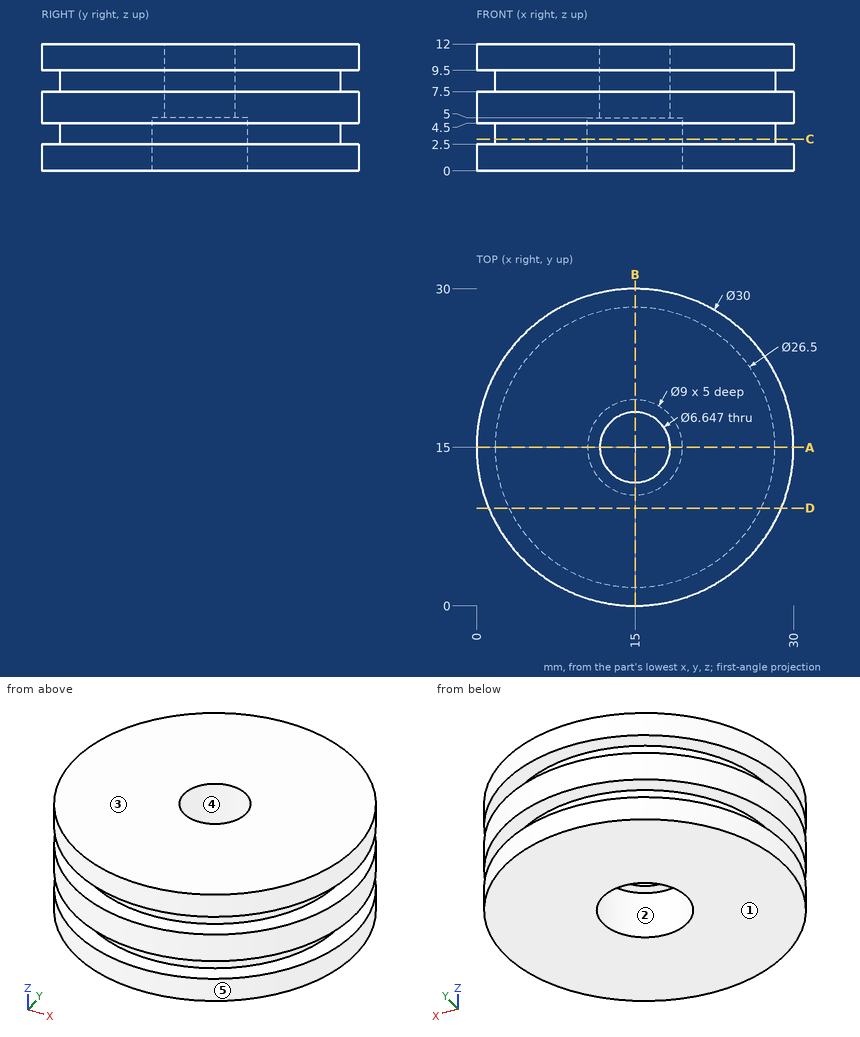
Check sheet for the drawn part. Datum: minimum x, y, z corner. Units: mm. A direction names the side the tool comes from. Give positions to 0.01 mm unless a question says otherwise; leave off trailing zeros. Loops run counter-clockwise (first coordinate to the right, second up) from the corner with the lowest first, then second, coordinate; pieces in that order, holes last. Notation, with made-up numbers: M 7,60 L 27,60 A20 ccw 27,70 Z; hole C -21,-13 d2. An arc over 180 degrees is marked long. Answer as CSV lines item,"result".
Item 1: Sectioned sample at D-D, the plane y = 9.25. Enter the section's corners in (x, z), then the cut area to 3 significant figures.
Reply:
outline,"M 1.15,0 L 28.85,0 L 28.85,2.5 L 26.94,2.5 L 26.94,4.5 L 28.85,4.5 L 28.85,7.5 L 26.94,7.5 L 26.94,9.5 L 28.85,9.5 L 28.85,12 L 1.15,12 L 1.15,9.5 L 3.06,9.5 L 3.06,7.5 L 1.15,7.5 L 1.15,4.5 L 3.06,4.5 L 3.06,2.5 L 1.15,2.5 Z"
area,"317 mm^2"
Item 2: Depth check by flat-ended pin: pin 1 Ø5.5 at (x, y) = (15, 15) entering from +Z; pin 2 Ø4.5 at (x, y) = (16.5, 16) entering from -Z; pin 3 Ø5 at (x, z) = (4.5, 4) entering from -Y; pin 4 Ø5 at (x, z) = (9.5, 3.5) entering from -Y. Enter the tip coordinate at first touch or a pass-through.
Reply:
pin 1,"through"
pin 2,"z = 5"
pin 3,"y = 2.34"
pin 4,"y = 0.35"
Item 3: Set-up check for the marked faces 1 and 2: record each of +Z, -Z, +X, -X, +Y, -Y from which the full face is reachable in a straight line by a thin tool's end or side.
Reply:
face 1,"-Z, +X, -X, +Y, -Y"
face 2,"-Z"
Item 4: Sectioned sample at C-C, the plane z = 3. Enter the section's corners in (x, y).
Reply:
outline,"C 15,15 d26.5; hole C 15,15 d9"
Item 5: Scan lines: L1, parallel to Z at x = 6, y = 4; L2, parallel to Y at x = 15, z = 8; L3, parallel to Y at x = 15, z = 1.35. Record each from-to range of solid material in increasing order.
Reply:
L1,"0 to 2.5, 4.5 to 7.5, 9.5 to 12"
L2,"1.75 to 11.68, 18.32 to 28.25"
L3,"0 to 10.5, 19.5 to 30"
Item 6: Draft check along Y on the marked faces 3, 4 and 5. Enter one of: pulls with the +Y half, pulls with the -Y half, needs draft (parallel to the pull), parting line crosses it, or undercut.
Reply:
face 3,"needs draft"
face 4,"undercut"
face 5,"parting line crosses it"
Item 7: Sectioned sample at A-A, the plane y = 15. Enter the section's corners in (x, z).
Reply:
outline,"M 0,0 L 10.5,0 L 10.5,5 L 11.68,5 L 11.68,12 L 0,12 L 0,9.5 L 1.75,9.5 L 1.75,7.5 L 0,7.5 L 0,4.5 L 1.75,4.5 L 1.75,2.5 L 0,2.5 Z; M 18.32,5 L 19.5,5 L 19.5,0 L 30,0 L 30,2.5 L 28.25,2.5 L 28.25,4.5 L 30,4.5 L 30,7.5 L 28.25,7.5 L 28.25,9.5 L 30,9.5 L 30,12 L 18.32,12 Z"
